from build123d import *

# Parameters (mm, degrees)
SKETCH_1_W          = 58
SKETCH_1_H          = 63
EXTRUDE_1_DEPTH     = 60
SKETCH_3_W          = 43
SKETCH_3_H          = 57
CUT_EXTRUDE_1_DEPTH = 56
CUT_EXTRUDE_2_DEPTH = 64
SKETCH_5_W          = 58
SKETCH_5_H          = 63
EXTRUDE_2_DEPTH     = 20


with BuildPart() as part:
    # 草图1 → 凸台-拉伸1 (new body)
    with BuildSketch(Plane.XY):
        with Locations((-34.85212532, 1.584978346)):
            Rectangle(SKETCH_1_W, SKETCH_1_H)
    extrude(amount=EXTRUDE_1_DEPTH)

    # 草图3 → 切除-拉伸1 (cut)
    with BuildSketch(Plane.XY.offset(60)):
        with Locations((-42.35212532, 1.584978346)):
            Rectangle(SKETCH_3_W, SKETCH_3_H)
    extrude(amount=-CUT_EXTRUDE_1_DEPTH, mode=Mode.SUBTRACT)

    # 草图4 → 切除-拉伸2 (cut, through all)
    with BuildSketch(Plane.XZ.offset(29.915021654)):
        Polygon((-63.85212532, 60), (-63.85212532, 14.614911021), (-28.222040277, 60), align=None)
    extrude(amount=-CUT_EXTRUDE_2_DEPTH, mode=Mode.SUBTRACT)

    # 草图5 → 凸台-拉伸2 (add)
    with BuildSketch(Plane(origin=(0, 0, 0), x_dir=(-1, 0, 0), z_dir=(0, 0, -1))):
        with Locations((34.85212532, 1.584978346)):
            Rectangle(SKETCH_5_W, SKETCH_5_H)
    extrude(amount=EXTRUDE_2_DEPTH)


solid = part.part
Read the model definition and answer for the solid it produces. Units are mm, in the model's axes. A direction names the side the tool comes from. Round coordinates to 2 decimals unless told otherwise and drop trailing zeros. Write each loop counter-clockwise with the first axis right and the second up, starting at its lowest first coordinate (ties: lowest second). Pieces come first, ordered by that corner, then holes.
1. The part is cut by section A-A, the plane z = 6.5. Determine the outline of the cut face in (x, y).
2. The part is cut by section C-C, the plane x = -46. Determine the outline of the cut face in (y, z), then the cut area to 3 significant figures.
3. The part is cut by section B-B, the plane y = 24. Determine the outline of the cut face in (x, z), then the cut area to 3 significant figures.
4. Given pin 1 Ø21.5 at (x, y) = (-41, 9.5) entering from +Z; pin 2 Ø17 at (y, z) = (5.5, 27.5) entering from -X, each flat-ended and moving along its own axis, determine where each tip first touches the part or whether it passes through.
5. Straight lines are drawn through the part: L1, parallel to Y at x = -57, z = 5; L2, parallel to Z at x = -24, y = 30; L3, parallel to X at y = 15, z = 28.5. For each, find the intervals that lie inside material, in ascending order.
6. Determine the mould class of faces 3 (the face through (-28, 33.085, 12)), 4 (the face through (-63.852, 1, -6)), 5 (the face through (-20.852, 1, 32)), 6 (the face through (-28, -29.915, 12)) for opening direction Y: pulls with the +Y half, pulls with the -Y half, needs draft (parallel to the pull), parting line crosses it, or undercut.
7. Which of the six approach directions +Z, -Z, +X, -X, +Y, -Y give full straight-line access (tool end or side, diameter ignored) to faces 1 (the face through (-46.286, -28.436, 36.99)), 2 (the face through (-38, -26.915, 26))?
Values:
1. outline: (-63.85, -29.92) - (-5.85, -29.92) - (-5.85, 33.08) - (-63.85, 33.08) - (-63.85, 30.08) - (-20.85, 30.08) - (-20.85, -26.92) - (-63.85, -26.92) - close
2. outline: (-29.92, -20) - (33.08, -20) - (33.08, 37.35) - (30.08, 37.35) - (30.08, 4) - (-26.92, 4) - (-26.92, 37.35) - (-29.92, 37.35) - close
2. area: 1,710 mm2
3. outline: (-63.85, -20) - (-5.85, -20) - (-5.85, 60) - (-20.85, 60) - (-20.85, 4) - (-63.85, 4) - close
3. area: 2,230 mm2
4. pin 1: stops at z = 4
4. pin 2: stops at x = -20.85
5. L1: y = -29.92 to -26.92, 30.08 to 33.08
5. L2: z = -20 to 4
5. L3: x = -20.85 to -5.85
6. face 3: pulls with the +Y half
6. face 4: needs draft
6. face 5: undercut
6. face 6: pulls with the -Y half
7. face 1: +Z, -X, +Y, -Y
7. face 2: +Z, -X
